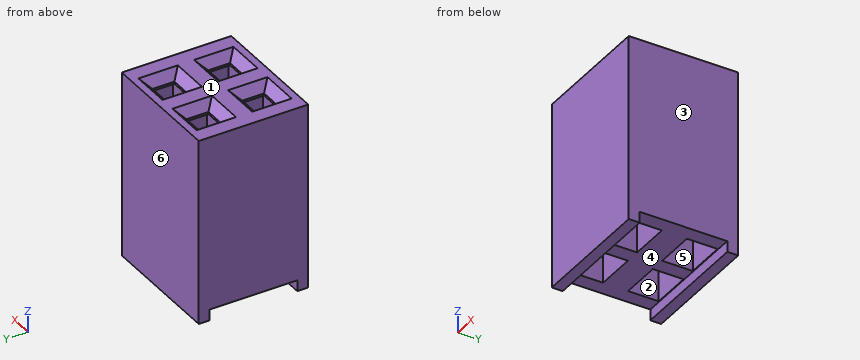
from build123d import *

# Parameters (mm, degrees)
SKETCH001_W      = 1.85
SKETCH001_H      = 1.4
EXTRUDE001_DEPTH = 8
SKETCH002_W      = 1
SKETCH002_H      = 1
EXTRUDE002_DEPTH = 9
SKETCH013_W      = 4
SKETCH013_H      = 4
EXTRUDE013_DEPTH = 0.5
SKETCH012_W      = 3.2
SKETCH012_H      = 5
EXTRUDE012_DEPTH = 8.5
CHAMFER003_SIZE  = 0.4
ARRAY006_X_COUNT = 2
ARRAY006_X_PITCH = 2.54


with BuildPart() as extrude001:
    # Sketch001 → Extrude001 (new body)
    with BuildSketch(Plane.XY):
        Rectangle(SKETCH001_W, SKETCH001_H)
    extrude(amount=EXTRUDE001_DEPTH)


with BuildPart() as fusion006:
    # Sketch002 → Extrude002 (new body)
    with BuildSketch(Plane.XY):
        Rectangle(SKETCH002_W, SKETCH002_H)
    extrude(amount=EXTRUDE002_DEPTH)

    # Fusion006: union Extrude001
    add(extrude001.part)


with BuildPart() as fusion006_1:
    # Fusion006 placement: moved
    add(fusion006.part.moved(Location((0, 1.27, 0))))


with BuildPart() as part_mirroring003:
    # Part__Mirroring003: instance of Fusion006
    add(fusion006_1.part.mirror(Plane(origin=(0, 0, 0), x_dir=(1, 0, 0), z_dir=(0, 1, 0))))


with BuildPart() as fusion007:
    # Sketch013 → Extrude013 (new body)
    with BuildSketch(Plane.XY):
        Rectangle(SKETCH013_W, SKETCH013_H)
    extrude(amount=EXTRUDE013_DEPTH)

    # Fusion007: union Part__Mirroring003, Fusion006
    add(part_mirroring003.part)
    add(fusion006_1.part)


with BuildPart() as body003:
    # Sketch012 → Extrude012 (new body)
    with BuildSketch(Plane.XY):
        Rectangle(SKETCH012_W, SKETCH012_H)
    extrude(amount=EXTRUDE012_DEPTH)

    # Cut003: cut Fusion007
    add(fusion007.part, mode=Mode.SUBTRACT)

    # Chamfer003
    chamfer003_edges = [body003.edges().sort_by_distance(p)[0] for p in [
        (0, -0.77, 8.5),
        (-0.5, -1.27, 8.5),
        (0, -1.77, 8.5),
        (0.5, -1.27, 8.5),
        (0.5, 1.27, 8.5),
        (0, 1.77, 8.5),
        (-0.5, 1.27, 8.5),
        (0, 0.77, 8.5),
    ]]
    chamfer(chamfer003_edges, length=CHAMFER003_SIZE)

    # Array006 X: body003 ×2


with BuildPart() as body003_1:
    add(body003.part)
    with Locations(*[(i * ARRAY006_X_PITCH, 0, 0) for i in range(1, ARRAY006_X_COUNT)]):
        add(body003.part)


solid = body003_1.part
Could you check a few things on this model? Use its own coordinates, in mm. Face numbers are marked on the shaded views. A direction names the side the tool comes from. Round coordinates to 2 decimals unless told otherwise and drop trailing zeros. Order: outer loops, then holes, each group sorted by start corner. A loop starts at its lowest first (then second) coordinate and runs counter-clockwise, first axis right, second up.
(1) Which directions (+Z, -Z, +X, -X, +Y, -Y) give clear straight access to the entire face, cutting with the end or side of a thin tool? Please do the marked faces 4, 5 and 6.
Response values:
face 4: -Z, +X, -X
face 5: -Z
face 6: +Z, -Z, +X, -X, +Y
(2) I'm going to push a flat-ended pin straight in: pin 1 (1.5 mm diameter, centred on x = 0, y = -1, fed in from -Z). Where does the tip first touch, or does it pass through?
Response values:
pin 1: stops at z = 0.5
(3) Imagine slicing it at D-D (y = -0.2). Write out the boundary of the cut face in (x, z).
Response values:
outline: (-1.6, 0.5) - (4.14, 0.5) - (4.14, 8.5) - (-1.6, 8.5) - close
(4) If we mould it in two halves opening along X, with no side actions, what happens to the marked faces 1, 2 and 3? For each: released by +X, released by -X, zero draft, split by the parting line, or undercut.
Response values:
face 1: zero draft
face 2: undercut
face 3: released by +X
(5) Imagine slicing it at A-A (x = 2.6). Count the separate pieces of the cut face and the enclosed holes in it, plus the area to 3 significant figures.
Response values:
separate pieces: 3
enclosed holes: 0
area: 18.2 mm2
(6) Imagine slicing it at B-B (y = 1.3). Write out the boundary of the cut face in (x, z) (3 decimals).
Response values:
outline: (-1.6, 0.5) - (-0.925, 0.5) - (-0.925, 8) - (-0.5, 8) - (-0.5, 8.1) - (-0.9, 8.5) - (-1.6, 8.5) - close; (0.5, 8) - (0.925, 8) - (0.925, 0.5) - (1.615, 0.5) - (1.615, 8) - (2.04, 8) - (2.04, 8.1) - (1.64, 8.5) - (0.9, 8.5) - (0.5, 8.1) - close; (3.04, 8) - (3.465, 8) - (3.465, 0.5) - (4.14, 0.5) - (4.14, 8.5) - (3.44, 8.5) - (3.04, 8.1) - close
(7) Please list where these lines run through material, in increasing order: line 1 along Y through (x, z) = (0.05, 6); line 2 along X through (y, z) = (1.4, 2.25) (3 decimals); line 3 along Z through (x, y) = (-1.05, 1.05).
Response values:
line 1: y = -2.5 to -1.97, -0.57 to 0.57, 1.97 to 2.5
line 2: x = -1.6 to -0.925, 0.925 to 1.615, 3.465 to 4.14
line 3: z = 0.5 to 8.5
(8) Imagine slicing it at C-C (z = 1.25). Write out the boundary of the cut face in (x, y) (3 decimals), plus the area to 3 significant figures.
Response values:
outline: (-1.6, -2.5) - (4.14, -2.5) - (4.14, 2.5) - (-1.6, 2.5) - close; hole (-0.925, -1.97) - (0.925, -1.97) - (0.925, -0.57) - (-0.925, -0.57) - close; hole (-0.925, 0.57) - (0.925, 0.57) - (0.925, 1.97) - (-0.925, 1.97) - close; hole (1.615, -1.97) - (3.465, -1.97) - (3.465, -0.57) - (1.615, -0.57) - close; hole (1.615, 0.57) - (3.465, 0.57) - (3.465, 1.97) - (1.615, 1.97) - close
area: 18.3 mm2
